from build123d import *

# Parameters (mm, degrees)
SKETCH1_R               = 4.5
SKETCH1_R_2             = 1.25
BOSS_EXTRUDE1_DEPTH     = 8
SKETCH2_R               = 1.75
SKETCH2_R_2             = 1.25
CUT_EXTRUDE1_DEPTH      = 4
SKETCH4_W               = 12
SKETCH4_H               = 12
SKETCH4_W_2             = 6.5
SKETCH4_H_2             = 6.5
BOSS_EXTRUDE2_DEPTH     = 15
SKETCH5_W               = 15
SKETCH5_H               = 12
BOSS_EXTRUDE3_DEPTH     = 8
CUT_EXTRUDE2_DEPTH      = 24.769728648
CUT_EXTRUDE2_DEPTH_BACK = 24.769728648
SKETCH6_R               = 1.1
FILLET1_R               = 2
SKETCH1_2_R             = 4.5
SKETCH1_2_R_2           = 1.25
CUT_EXTRUDE5_DEPTH      = 8
BOSS_EXTRUDE5_OUTLINE_W = 6.5
BOSS_EXTRUDE5_OUTLINE_H = 6.5
BOSS_EXTRUDE5_OUTLINE_R = 1.75
BOSS_EXTRUDE5_DEPTH     = 3


# Read off the part's stored shape, not the designer's step: Boss-Extrude5
with BuildPart() as part:
    # Sketch1 → Boss-Extrude1 (new body)
    with BuildSketch(Plane.XY):
        Circle(SKETCH1_R)
        Circle(SKETCH1_R_2, mode=Mode.SUBTRACT)
    extrude(amount=BOSS_EXTRUDE1_DEPTH)

    # Sketch2 → Cut-Extrude1 (cut)
    with BuildSketch(Plane(origin=(0, 0, 0), x_dir=(-1, 0, 0), z_dir=(0, 0, -1))):
        Circle(SKETCH2_R)
        Circle(SKETCH2_R_2, mode=Mode.SUBTRACT)
    extrude(amount=-CUT_EXTRUDE1_DEPTH, mode=Mode.SUBTRACT)

    # Sketch4 → Boss-Extrude2 (add)
    with BuildSketch(Plane(origin=(0, 0, 0), x_dir=(-1, 0, 0), z_dir=(0, 0, -1))):
        Rectangle(SKETCH4_W, SKETCH4_H)
        Rectangle(SKETCH4_W_2, SKETCH4_H_2, mode=Mode.SUBTRACT)
    extrude(amount=BOSS_EXTRUDE2_DEPTH)

    # Sketch5 → Boss-Extrude3 (add)
    with BuildSketch(Plane(origin=(6, 0, 0), x_dir=(0, 0, -1), z_dir=(1, 0, 0))):
        with Locations((7.5, 0)):
            Rectangle(SKETCH5_W, SKETCH5_H)
    extrude(amount=BOSS_EXTRUDE3_DEPTH)

    # Sketch6 → Cut-Extrude2 (cut, two sides: drawn at the far end of the back side and taken through both)
    with BuildSketch(Plane(origin=(0, 6, 0), x_dir=(1, 0, 0), z_dir=(0, 1, 0)).offset(-CUT_EXTRUDE2_DEPTH_BACK)):
        with Locations(Location((9, 11.25, 0), (0, 0, 270))):
            Circle(SKETCH6_R)
        with Locations(Location((9, 5, 0), (0, 0, 270))):
            Circle(SKETCH6_R)
    extrude(amount=CUT_EXTRUDE2_DEPTH + CUT_EXTRUDE2_DEPTH_BACK, mode=Mode.SUBTRACT)

    # Fillet1
    fillet1_edges = [part.edges().sort_by_distance(p)[0] for p in [
        (-6, -6, -7.5),
        (-6, 6, -7.5),
        (14, 6, -7.5),
        (14, -6, -7.5),
    ]]
    fillet(fillet1_edges, radius=FILLET1_R)

    # Sketch1<2> → Cut-Extrude5 (cut)
    with BuildSketch(Plane.XY):
        Circle(SKETCH1_2_R)
        Circle(SKETCH1_2_R_2, mode=Mode.SUBTRACT)
    extrude(amount=CUT_EXTRUDE5_DEPTH, mode=Mode.SUBTRACT)

    # Boss-Extrude5 outline → Boss-Extrude5 (add)
    with BuildSketch(Plane(origin=(0, 0, 0), x_dir=(-1, 0, 0), z_dir=(0, 0, -1))):
        Rectangle(BOSS_EXTRUDE5_OUTLINE_W, BOSS_EXTRUDE5_OUTLINE_H)
        Circle(BOSS_EXTRUDE5_OUTLINE_R, mode=Mode.SUBTRACT)
    extrude(amount=BOSS_EXTRUDE5_DEPTH)


solid = part.part
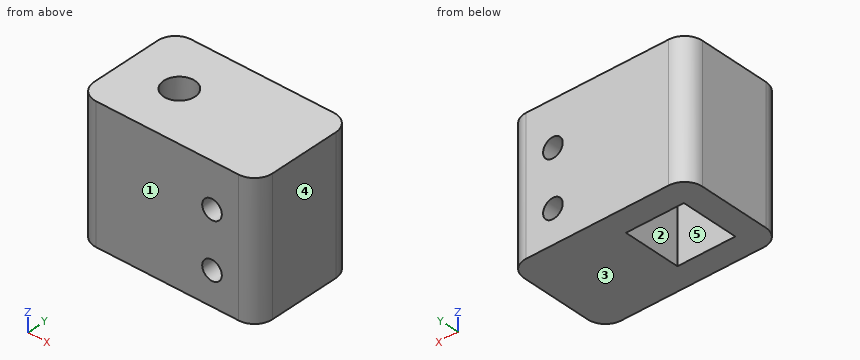
Could you check a few things on this model? Use its own coordinates, in mm. Face numbers are marked on the shaded views. A direction names the side the tool comes from. Give positions to 0.01 mm unless a question says otherwise; leave off trailing zeros. Write each loop counter-clockwise with the first axis right and the second up, starting at its lowest first coordinate (ties: lowest second). Pieces come first, ordered by that corner, then holes. Notation, with made-up numbers: (0.5, 24) -> (58.5, 24) arc R23 ccw to (58.5, 62) -> close; hole circle Ø4 at (48, -31). An arc over 180 degrees is marked (long way). Write each question's results on one line, items separated by ' | '. Start each with the question number.
Q1. I'm going to push a flat-ended pin straight in: pin 1 Ø3 at (x, y) = (0, 0) entering from +Z. Where does the tip first touch, or does it pass through?
Q2. Suppose I cut it at B-B, the plane z = -11.25. List the corners of the cut face in (x, y) for me, and give its area (3 significant figures).
Q3. Suppose I cut it at C-C, the plane z = -2. List the corners of the cut face in (x, y) for me.
Q4. I need wall thicknesses on probe 1 along Z at (x, y) = (9, 0); probe 2 along X at (y, z) = (2.25, -11.25); probe 3 along X at (y, z) = (-1.75, -9.25). Which ranges of each line are inside material? Lowest first, please.
Q5. Suppose I cut it at A-A, the plane y = 0. List the corners of the cut face in (x, z) for me, and give its area (3 significant figures).
Q6. We'd pull the mould along X, two halves only. Please class the marked faces 3, 4 and 5: +X half, -X half, draft (parallel to the pull), parting line (faces both ways), or undercut.
Q7. Suppose I cut it at D-D, the plane x = 0. List the corners of the cut face in (y, z) for me, and give its area (3 significant figures).
Q8. Which directions (+Z, -Z, +X, -X, +Y, -Y) give clear straight access to the entire face, cutting with the end or side of a thin tool? Please do the marked faces 1 and 2.
Outcome:
1) pin 1: through
2) outline: (-6, -4) arc R2 ccw to (-4, -6) -> (7.9, -6) -> (7.9, 6) -> (-4, 6) arc R2 ccw to (-6, 4) -> close; (10.1, -6) -> (12, -6) arc R2 ccw to (14, -4) -> (14, 4) arc R2 ccw to (12, 6) -> (10.1, 6) -> close; hole (-3.25, -3.25) -> (3.25, -3.25) -> (3.25, 3.25) -> (-3.25, 3.25) -> close | area: 168 mm2
3) outline: (-6, -4) arc R2 ccw to (-4, -6) -> (12, -6) arc R2 ccw to (14, -4) -> (14, 4) arc R2 ccw to (12, 6) -> (-4, 6) arc R2 ccw to (-6, 4) -> close; hole circle Ø3.5 at (0, 0)
4) probe 1: -15 to -12.35, -10.15 to -6.1, -3.9 to 0 | probe 2: -6 to -3.25, 3.25 to 7.9, 10.1 to 14 | probe 3: -6 to -3.25, 3.25 to 14
5) outline: (-6, -15) -> (-3.25, -15) -> (-3.25, -3) -> (-1.75, -3) -> (-1.75, 0) -> (-6, 0) -> close; (1.75, -3) -> (3.25, -3) -> (3.25, -15) -> (14, -15) -> (14, 0) -> (1.75, 0) -> close; hole circle Ø2.2 at (9, -11.25); hole circle Ø2.2 at (9, -5) | area: 204 mm2
6) face 3: draft | face 4: +X half | face 5: undercut
7) outline: (-6, -15) -> (-3.25, -15) -> (-3.25, -3) -> (-1.75, -3) -> (-1.75, 0) -> (-6, 0) -> close; (1.75, -3) -> (3.25, -3) -> (3.25, -15) -> (6, -15) -> (6, 0) -> (1.75, 0) -> close | area: 91.5 mm2
8) face 1: +Z, -Z, +X, -X, -Y | face 2: -Z
